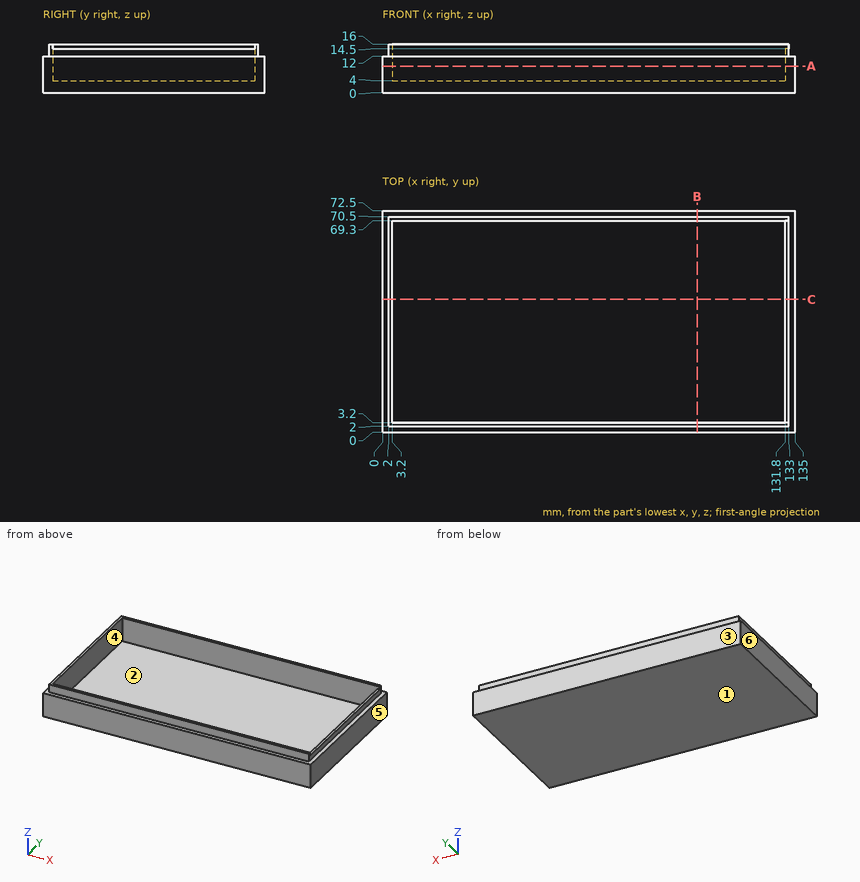
Here's the drawing with two shaded views (mm, measured from the low corner). I have some questions. A direction names the side the tool comes from. Give positions to 0.01 mm unless a question says otherwise; leave off trailing zeros. Write each loop counter-clockwise with the first axis right and the second up, starting at its lowest first coordinate (ties: lowest second). Pieces come first, ordered by that corner, then holes. Notation, with made-up numbers: (-8, -39.5) -> (28, -39.5) arc R7 ccw to (28, -28.5) -> close; hole circle Ø7 at (46.5, -5). An arc over 180 degrees is marked (long way). Answer as a JSON object with one key per item and string values. Group by question number.
Item 1: Please list where these lines run through material, in increasing order: line 1 (X direction, y = 24.5, z = 5.5); line 2 (Y direction, x = 124, z = 11.75); line 3 (Y direction, x = 6, z = 14.5). Write a range as [from, to].
Item 2: We'd pull the mould along X, two halves only. Please class the marked faces 3, 4, 5 and 6: +X half, -X half, draft (parallel to the pull), parting line (faces both ways), or undercut.
Item 3: Suppose I cut it at B-B (x = 103). Please give me the cut outline in (y, z), plus the area to 3 significant figures.
Item 4: For the marked faces 1 and 2, which set-ups out of +Z, -Z, +X, -X, +Y, -Y let a thin tool reach every point of the face, with its end or its side?
Item 5: Suppose I cut it at A-A (z = 8.75). Please give me the cut outline in (x, y).
Item 6: I'm going to push flat-ended pins straight in: P1, Ø22, axis at x = 97.5, y = 27, coming from the +Z side; P2, Ø1, axis at y = 64, z = 13.5, coming from the +X side; P3, Ø2, axis at x = 16.5, z = 14.5, coming from the -Y side. Where does each tip first touch, or does it pass through?
Item 7: Suppose I cut it at C-C (y = 43.5). Please give me the cut outline in (x, z), plus the area to 3 significant figures.
Findings:
{
 "1": {"line 1": "x = [0, 3.2], [131.8, 135]", "line 2": "y = [0, 3.2], [69.3, 72.5]", "line 3": "y = [2, 3.2], [69.3, 70.5]"},
 "2": {"face 3": "draft", "face 4": "undercut", "face 5": "+X half", "face 6": "-X half"},
 "3": {"outline": "(0, 0) -> (72.5, 0) -> (72.5, 12) -> (70.5, 12) -> (70.5, 16) -> (69.3, 16) -> (69.3, 4) -> (3.2, 4) -> (3.2, 16) -> (2, 16) -> (2, 12) -> (0, 12) -> close", "area": "351 mm²"},
 "4": {"face 1": "-Z, +X, -X, +Y, -Y", "face 2": "+Z"},
 "5": {"outline": "(0, 0) -> (135, 0) -> (135, 72.5) -> (0, 72.5) -> close; hole (3.2, 3.2) -> (131.8, 3.2) -> (131.8, 69.3) -> (3.2, 69.3) -> close"},
 "6": {"P1": "stops at z = 4", "P2": "stops at x = 133", "P3": "stops at y = 2"},
 "7": {"outline": "(0, 0) -> (135, 0) -> (135, 12) -> (133, 12) -> (133, 14.5) -> (131.8, 14.5) -> (131.8, 4) -> (3.2, 4) -> (3.2, 16) -> (2, 16) -> (2, 12) -> (0, 12) -> close", "area": "599 mm²"}
}
